from build123d import *

# Parameters (mm, degrees)
F0_W      = 152.605712
F0_H      = 152.340234
F1_DEPTH  = 46.228
F2_R      = 55.88
F3_R      = 55.88
F4_R      = 55.88
F5_R      = 55.88
F6_W      = 103.709646
F6_H      = 110.155954
F6_W_2    = 66.169404
F6_H_2    = 74.132488
F7_DEPTH  = 25.4
F8_R      = 24.52841
F9_R      = 9.811364
F10_R     = 23.330853
F11_DEPTH = 25.4
F12_R     = 6.759077
F13_DEPTH = 25.4
F14_R     = 5.952934
F15_DEPTH = 62.484


with BuildPart() as f1:
    # F0 (on Top) → F1 (new body)
    with BuildSketch(Plane.XY):
        Rectangle(F0_W, F0_H)
    extrude(amount=F1_DEPTH)

    # F2
    f2_edges = [f1.edges().sort_by_distance(p)[0] for p in [
        (76.302856, 76.170117, 23.114),
    ]]
    fillet(f2_edges, radius=F2_R)

    # F3
    f3_edges = [f1.edges().sort_by_distance(p)[0] for p in [
        (-76.302856, 76.170117, 23.114),
    ]]
    fillet(f3_edges, radius=F3_R)

    # F4
    f4_edges = [f1.edges().sort_by_distance(p)[0] for p in [
        (-76.302856, -76.170117, 23.114),
    ]]
    fillet(f4_edges, radius=F4_R)

    # F5
    f5_edges = [f1.edges().sort_by_distance(p)[0] for p in [
        (76.302856, -76.170117, 23.114),
    ]]
    fillet(f5_edges, radius=F5_R)

    # F6 (on face) → F7 (cut)
    with BuildSketch(Plane.XY.offset(46.228)):
        Rectangle(F6_W, F6_H)
        Rectangle(F6_W_2, F6_H_2, mode=Mode.SUBTRACT)
    extrude(amount=-F7_DEPTH, mode=Mode.SUBTRACT)

    # F8
    f8_edges = [f1.edges().sort_by_distance(p)[0] for p in [
        (-51.854823, -55.077977, 33.528),
        (51.854823, -55.077977, 33.528),
        (51.854823, 55.077977, 33.528),
        (-51.854823, 55.077977, 33.528),
    ]]
    fillet(f8_edges, radius=F8_R)

    # F9
    f9_edges = [f1.edges().sort_by_distance(p)[0] for p in [
        (-33.084702, -37.066244, 33.528),
        (-33.084702, 37.066244, 33.528),
        (33.084702, 37.066244, 33.528),
        (33.084702, -37.066244, 33.528),
    ]]
    fillet(f9_edges, radius=F9_R)

    # F10 (on face) → F11 (cut)
    with BuildSketch(Plane.XY.offset(46.228)):
        Circle(F10_R)
    extrude(amount=-F11_DEPTH, mode=Mode.SUBTRACT)

    # F12 (on face) → F13 (cut)
    with BuildSketch(Plane.XY.offset(46.228)):
        with Locations((23.273338, 27.25488)):
            Circle(F12_R)
    extrude(amount=-F13_DEPTH, mode=Mode.SUBTRACT)

    # F14 (on face) → F15 (cut)
    with BuildSketch(Plane.XY.offset(46.228)):
        with Locations((44.878781, 59.487075)):
            Circle(F14_R)
    extrude(amount=-F15_DEPTH, mode=Mode.SUBTRACT)


solid = f1.part
Could you check a few things on this model? Use its own coordinates, in mm. A direction names the side the tool comes from. Give positions to 0.01 mm unless a question says otherwise; leave off trailing zeros. Order: outer loops, then holes, each group sorted by start corner. A loop starts at its lowest first (then second) coordinate and runs counter-clockwise, first axis right, second up. Notation, with made-up numbers: (20, -34.5) - (40, -34.5) arc R25 cw to (40, -19.5) - close; hole circle Ø1 at (13.5, 87). An arc over 180 degrees is marked (long way). One line per item, written item: value. Start each with the question number.
1. Imagine slicing it at A-A on z = 28. List the corners of the cut face in (x, y) for me, plus the area to 3 significant figures.
2. Imagine slicing it at B-B on x = 0. List the corners of the cut face in (y, z) for me.
3. Imagine slicing it at D-D on z = 5. List the corners of the cut face in (x, y) for me, plus the area to 3 significant figures.
4. If I drill on probe 1 along Y at (x, z) = (0, 40); probe 2 along X at (y, z) = (-24.5, 26); probe 3 along X at (y, z) = (32.5, 24) (3 decimals), over which ranges is the centre line in solid material (lowest first)?
5. For faces 1 (the face through (-23, -8, 46.228)), 2 (the face through (-30.1, -34.3, 33.4)), which set-ups out of +Z, -Z, +X, -X, +Y, -Y let a thin tool reach every point of the face, with its end or its side?
6. Thinking about a two-plate mould opening in X: for faces 3 (the face through (44.86, 47.7, 33.35)), 4 (the face through (0, -76.17, 23)), 5 (the face through (30.1, -34.3, 33.4)), 6 (the face through (60.368, 59.366, 23.438)), which applies, +X half, -X half, draft (parallel to the pull), parting line (faces both ways), or undercut?
7. Imagine slicing it at C-C on y = 0. List the corners of the cut face in (x, z) for me.
8. For P1, Ø3, axis at x = 56, z = 12, coming from the +Y side; P2, Ø5, axis at y = 47.5, z = 15, coming from the -X side; P3, Ø1.5, axis at x = -54, z = 9, coming from the +Y side, each with a flat end and sliding along its axis, tell me the tip position at first contact or that it passes through.
Values:
1. outline: (-76.3, -20.29) arc R55.88 ccw to (-20.42, -76.17) - (20.42, -76.17) arc R55.88 ccw to (76.3, -20.29) - (76.3, 20.29) arc R55.88 ccw to (20.42, 76.17) - (-20.42, 76.17) arc R55.88 ccw to (-76.3, 20.29) - close; (-33.08, -27.25) arc R9.81 ccw to (-23.27, -37.07) - (23.27, -37.07) arc R9.81 ccw to (33.08, -27.25) - (33.08, 27.25) arc R9.81 ccw to (23.27, 37.07) - (-23.27, 37.07) arc R9.81 ccw to (-33.08, 27.25) - close; hole (-51.85, -30.55) arc R24.53 ccw to (-27.33, -55.08) - (27.33, -55.08) arc R24.53 ccw to (51.85, -30.55) - (51.85, 30.55) arc R24.53 ccw to (27.33, 55.08) - (-27.33, 55.08) arc R24.53 ccw to (-51.85, 30.55) - close; hole circle Ø46.66 at (0, 0); hole circle Ø13.52 at (23.27, 27.25); hole circle Ø11.91 at (44.88, 59.49)
1. area: 12,500 mm²
2. outline: (-76.17, 0) - (76.17, 0) - (76.17, 46.23) - (55.08, 46.23) - (55.08, 20.83) - (37.07, 20.83) - (37.07, 46.23) - (23.33, 46.23) - (23.33, 20.83) - (-23.33, 20.83) - (-23.33, 46.23) - (-37.07, 46.23) - (-37.07, 20.83) - (-55.08, 20.83) - (-55.08, 46.23) - (-76.17, 46.23) - close
3. outline: (-76.3, -20.29) arc R55.88 ccw to (-20.42, -76.17) - (20.42, -76.17) arc R55.88 ccw to (76.3, -20.29) - (76.3, 20.29) arc R55.88 ccw to (20.42, 76.17) - (-20.42, 76.17) arc R55.88 ccw to (-76.3, 20.29) - close; hole circle Ø11.91 at (44.88, 59.49)
3. area: 20,500 mm²
4. probe 1: -76.17 to -55.08, -37.07 to -23.33, 23.33 to 37.07, 55.08 to 76.17
4. probe 2: -76.14 to -51.85, -33.08 to 33.08, 51.85 to 76.14
4. probe 3: -74.953 to -51.777, -31.565 to 19.01, 27.536 to 31.565, 51.777 to 74.953
5. face 1: +Z, +X, -X, +Y, -Y
5. face 2: +Z
6. face 3: undercut
6. face 4: draft
6. face 5: undercut
6. face 6: +X half
7. outline: (-76.3, 0) - (76.3, 0) - (76.3, 46.23) - (51.85, 46.23) - (51.85, 20.83) - (33.08, 20.83) - (33.08, 46.23) - (23.33, 46.23) - (23.33, 20.83) - (-23.33, 20.83) - (-23.33, 46.23) - (-33.08, 46.23) - (-33.08, 20.83) - (-51.85, 20.83) - (-51.85, 46.23) - (-76.3, 46.23) - close
8. P1: y = 64.58
8. P2: x = -70.54
8. P3: y = 65.51
